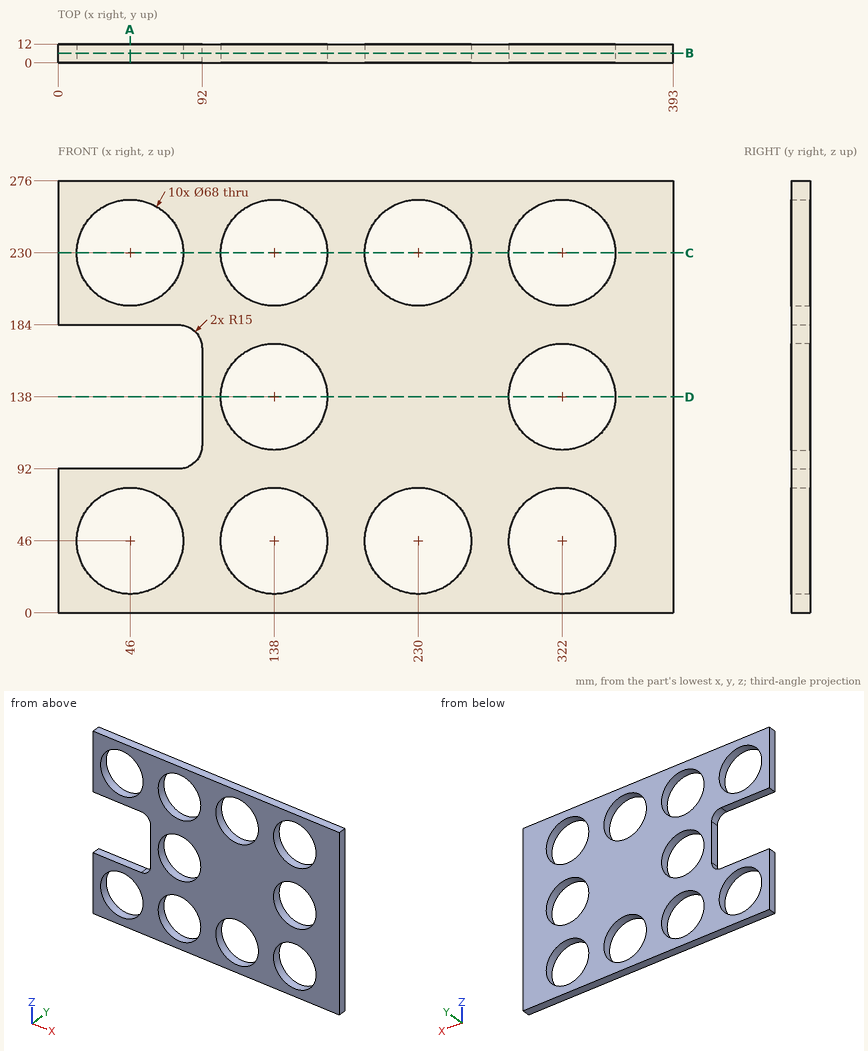
Verification items for this drawing (mm, ordinates from the low corner). Round coordinates to 2 decimals unless told otherwise and drop trailing zeros. Loops run counter-clockwise (first coordinate to the right, second up) from the corner with the lowest first, then second, coordinate; pieces in that order, holes last. Notation, with made-up numbers: (26, -3.5) -> (48, -3.5) arc R24 cw to (48, 12.5) -> close; hole circle Ø8 at (-16.5, 49.5). An arc over 180 degrees is marked (long way). Write item = value, one per line. Start each with the question number.
1) Sectioned sample at B-B, the plane y = 6.25. State how many separate pieces and enclosed holes the cut face has, plus the area to 3 significant figures.
2) Sectioned sample at A-A, the plane x = 46. Record the cut outline in (y, z).
3) Thickness scan on probe 1 along X at (y, z) = (9.25, 230); probe 2 along Z at (x, y) = (18.5, 1.75); probe 3 along X at (y, z) = (9.75, 120.5). Record the ranges inside material, lowest first.
4) Sectioned sample at D-D, the plane z = 138. Record the cut outline in (x, y), plus the area to 3 significant figures.
5) Sectioned sample at C-C, the plane z = 230. Record the cut outline in (x, y).
Results are:
q1.separate_pieces = 1
q1.enclosed_holes = 10
q1.area = 63,800 mm^2
q2.outline = (0, 0) -> (12, 0) -> (12, 12) -> (0, 12) -> close; (0, 80) -> (12, 80) -> (12, 92) -> (0, 92) -> close; (0, 184) -> (12, 184) -> (12, 196) -> (0, 196) -> close; (0, 264) -> (12, 264) -> (12, 276) -> (0, 276) -> close
q3.probe_1 = 0 to 12, 80 to 104, 172 to 196, 264 to 288, 356 to 393
q3.probe_2 = 0 to 26.01, 65.99 to 92, 184 to 210.01, 249.99 to 276
q3.probe_3 = 92 to 108.85, 167.15 to 292.85, 351.15 to 393
q4.outline = (92, 0) -> (104, 0) -> (104, 12) -> (92, 12) -> close; (172, 0) -> (288, 0) -> (288, 12) -> (172, 12) -> close; (356, 0) -> (393, 0) -> (393, 12) -> (356, 12) -> close
q4.area = 1,980 mm^2
q5.outline = (0, 0) -> (12, 0) -> (12, 12) -> (0, 12) -> close; (80, 0) -> (104, 0) -> (104, 12) -> (80, 12) -> close; (172, 0) -> (196, 0) -> (196, 12) -> (172, 12) -> close; (264, 0) -> (288, 0) -> (288, 12) -> (264, 12) -> close; (356, 0) -> (393, 0) -> (393, 12) -> (356, 12) -> close
